from build123d import *

# Parameters (mm, degrees)
SKETCH1_R           = 1.75
BOSS_EXTRUDE1_DEPTH = 8
SKETCH2_R           = 3
CUT_EXTRUDE1_DEPTH  = 1.4
CUT_EXTRUDE2_DEPTH  = 59.268773799
FILLET1_R           = 2
CHAMFER1_SIZE       = 1
SKETCH4_R           = 4.541609358
CUT_EXTRUDE3_DEPTH  = 59.268773799
CHAMFER2_SIZE       = 2


with BuildPart() as part:
    # Sketch1 → Boss-Extrude1 (new body)
    with BuildSketch(Plane(origin=(0, 0, 0), x_dir=(1, 0, 0), z_dir=(0, 1, 0))):
        with BuildLine():
            Line((4.375, 16.94430214), (51.25, 4.841229183))
            ThreePointArc((51.25, 4.841229183), (55, 0), (51.25, -4.841229183))
            Line((51.25, -4.841229183), (4.375, -16.94430214))
            ThreePointArc((4.375, -16.94430214), (-17.5, 0), (4.375, 16.94430214))
        make_face()
        with Locations(Location((6.75, 11.691342951, 0), (0, 0, 270))):
            Circle(SKETCH1_R, mode=Mode.SUBTRACT)
        with Locations(Location((-13.5, 0, 0), (0, 0, 270))):
            Circle(SKETCH1_R, mode=Mode.SUBTRACT)
        with Locations(Location((6.75, -11.691342951, 0), (0, 0, 270))):
            Circle(SKETCH1_R, mode=Mode.SUBTRACT)
    extrude(amount=BOSS_EXTRUDE1_DEPTH)

    # Sketch2 → Cut-Extrude1 (cut)
    with BuildSketch(Plane(origin=(0, 8, 0), x_dir=(1, 0, 0), z_dir=(0, 1, 0))):
        with Locations(Location((6.75, -11.691342951, 0), (0, 0, 270))):
            Circle(SKETCH2_R)
        with Locations(Location((6.75, 11.691342951, 0), (0, 0, 270))):
            Circle(SKETCH2_R)
        with Locations(Location((-13.5, 0, 0), (0, 0, 270))):
            Circle(SKETCH2_R)
    extrude(amount=-CUT_EXTRUDE1_DEPTH, mode=Mode.SUBTRACT)

    # Sketch3 → Cut-Extrude2 (cut, through all)
    with BuildSketch(Plane(origin=(0, 8, 0), x_dir=(1, 0, 0), z_dir=(0, 1, 0))):
        with BuildLine():
            Line((21.175820833, -6.4095755), (46, 0))
            Line((46, 0), (21.175820833, 6.4095755))
            ThreePointArc((21.175820833, 6.4095755), (22.124602732, 0), (21.175820833, -6.4095755))
        make_face()
    extrude(amount=-CUT_EXTRUDE2_DEPTH, mode=Mode.SUBTRACT)

    # Fillet1
    fillet1_edges = [part.edges().sort_by_distance(p)[0] for p in [
        (21.175820833, 4, 6.4095755),
        (21.175820833, 4, -6.4095755),
        (46, 4, 0),
    ]]
    fillet(fillet1_edges, radius=FILLET1_R)

    # Chamfer1
    chamfer1_edges = [part.edges().sort_by_distance(p)[0] for p in [
        (6.75, 6.6, 8.691342951),
        (6.75, 6.6, -14.691342951),
        (-13.5, 6.6, -3),
    ]]
    chamfer(chamfer1_edges, length=CHAMFER1_SIZE)

    # Sketch4 → Cut-Extrude3 (cut, through all)
    with BuildSketch(Plane(origin=(0, 8, 0), x_dir=(1, 0, 0), z_dir=(0, 1, 0))):
        with Locations(Location((0, 0, 0), (0, 0, 270))):
            Circle(SKETCH4_R)
    extrude(amount=-CUT_EXTRUDE3_DEPTH, mode=Mode.SUBTRACT)

    # Chamfer2
    # the kernel refuses this chamfer: 2 mm, written as the material it takes off along each edge
    with BuildSketch(Plane(origin=(38, 0, 0), x_dir=(0.25, 0, 0.9682458365518543), z_dir=(-0.9682458365518543, 0, 0.25))) as chamfer2_piece_1:
        Polygon((2 + CHAMFER2_SIZE, 0), (2, CHAMFER2_SIZE), (2, 0), align=None)
    revolve(axis=Axis((38, 0, 0), (0, 1, 0)), revolution_arc=151.044975628, mode=Mode.SUBTRACT)
    with BuildSketch(Plane(origin=(24.346197065, 0, -5.590987877), x_dir=(0.24990547922782413, -0.027495876610586372, -0.9678797591753465), z_dir=(0.9682458365518543, 0, 0.24999999999999997)), Plane(origin=(38.5, 0, 1.936491673), x_dir=(0.2499054792278243, -0.027495876610585942, 0.9678797591753466), z_dir=(-0.9682458365518543, 0, 0.2500000000000001)), Plane(origin=(38.5, 8, -1.936491673), x_dir=(0.24990547922782413, 0.027495876610586497, -0.9678797591753466), z_dir=(-0.9682458365518543, 0, -0.24999999999999997)), Plane(origin=(24.346197065, 8, 5.590987877), x_dir=(0.2499054792278243, 0.02749587661058648, 0.9678797591753466), z_dir=(0.9682458365518543, 0, -0.2500000000000001))) as chamfer2_piece_2:
        Polygon((CHAMFER2_SIZE * 0.999621916911, CHAMFER2_SIZE * 0.0274958766106), (-CHAMFER2_SIZE * 0.0274958766106, CHAMFER2_SIZE * 0.999621916911), (0, 0), align=None)
    extrude(amount=14.617984814, mode=Mode.SUBTRACT)
    with BuildSketch(Plane(origin=(23.846197065, 0, -3.654496203), x_dir=(-0.9884596787014585, 0, 0.15148420241533292), z_dir=(0.15148420241533292, 0, 0.9884596787014585))) as chamfer2_piece_3:
        Polygon((2 + CHAMFER2_SIZE, 0), (2, -CHAMFER2_SIZE), (2, 0), align=None)
    revolve(axis=Axis((23.846197065, 0, -3.654496203), (0, -1, 0)), revolution_arc=113.190460245, mode=Mode.SUBTRACT)
    with BuildSketch(Plane(origin=(23.846197065, 0, 3.654496203), x_dir=(0.25000000000000006, 0, 0.9682458365518543), z_dir=(0.9682458365518543, 0, -0.25000000000000006))) as chamfer2_piece_4:
        Polygon((2 + CHAMFER2_SIZE, 0), (2, -CHAMFER2_SIZE), (2, 0), align=None)
    revolve(axis=Axis((23.846197065, 0, 3.654496203), (0, -1, 0)), revolution_arc=113.190460245, mode=Mode.SUBTRACT)
    with BuildSketch(Plane(origin=(0, 0, 0), x_dir=(0.988459678701458, 0, 0.151484202415335), z_dir=(-0.151484202415335, 0, 0.988459678701458))) as chamfer2_piece_5:
        Polygon((22.124602732 - CHAMFER2_SIZE, 0), (22.124602732, CHAMFER2_SIZE), (22.124602732, 0), align=None)
    revolve(axis=Axis((0, 0, 0), (0, 1, 0)), revolution_arc=17.425896117, mode=Mode.SUBTRACT)
    with BuildSketch(Plane(origin=(23.846197065, 8, -3.654496203), x_dir=(-0.9884596787014583, 0, 0.15148420241533467), z_dir=(0.15148420241533467, 0, 0.9884596787014583))) as chamfer2_piece_6:
        Polygon((2 + CHAMFER2_SIZE, 0), (2, CHAMFER2_SIZE), (2, 0), align=None)
    revolve(axis=Axis((23.846197065, 8, -3.654496203), (0, -1, 0)), revolution_arc=113.190460245, mode=Mode.SUBTRACT)
    with BuildSketch(Plane(origin=(0, 8, 0), x_dir=(0.9884596787014582, 0, -0.1514842024153346), z_dir=(-0.1514842024153346, 0, -0.9884596787014582))) as chamfer2_piece_7:
        Polygon((22.124602732 - CHAMFER2_SIZE, 0), (22.124602732, CHAMFER2_SIZE), (22.124602732, 0), align=None)
    revolve(axis=Axis((0, 8, 0), (0, -1, 0)), revolution_arc=17.425896117, mode=Mode.SUBTRACT)
    with BuildSketch(Plane(origin=(23.846197065, 8, 3.654496203), x_dir=(0.25000000000000006, 0, 0.9682458365518543), z_dir=(0.9682458365518543, 0, -0.25000000000000006))) as chamfer2_piece_8:
        Polygon((2 + CHAMFER2_SIZE, 0), (2, CHAMFER2_SIZE), (2, 0), align=None)
    revolve(axis=Axis((23.846197065, 8, 3.654496203), (0, -1, 0)), revolution_arc=113.190460245, mode=Mode.SUBTRACT)
    with BuildSketch(Plane(origin=(38, 8, 0), x_dir=(0.25, 0, 0.9682458365518543), z_dir=(-0.9682458365518543, 0, 0.25))) as chamfer2_piece_9:
        Polygon((2 + CHAMFER2_SIZE, 0), (2, -CHAMFER2_SIZE), (2, 0), align=None)
    revolve(axis=Axis((38, 8, 0), (0, 1, 0)), revolution_arc=151.044975628, mode=Mode.SUBTRACT)
    with BuildSketch(Plane(origin=(4.375, 0, -16.94430214), x_dir=(-0.24990547922782413, -0.027495876610586365, 0.9678797591753465), z_dir=(0.9682458365518543, 0, 0.24999999999999997)), Plane(origin=(51.25, 0, 4.841229183), x_dir=(-0.2499054792278242, -0.027495876610586348, -0.9678797591753466), z_dir=(-0.9682458365518543, 0, 0.24999999999999997))) as chamfer2_piece_10:
        Polygon((CHAMFER2_SIZE * 0.999621916911, -CHAMFER2_SIZE * 0.0274958766106), (-CHAMFER2_SIZE * 0.0274958766106, -CHAMFER2_SIZE * 0.999621916911), (0, 0), align=None)
    extrude(amount=48.412291828, mode=Mode.SUBTRACT)
    with BuildSketch(Plane(origin=(0, 0, 0), x_dir=(0.24999999999999994, 0, 0.9682458365518543), z_dir=(0.9682458365518543, 0, -0.24999999999999994))) as chamfer2_piece_11:
        Polygon((17.5 - CHAMFER2_SIZE, 0), (17.5, -CHAMFER2_SIZE), (17.5, 0), align=None)
    revolve(axis=Axis((0, 0, 0), (0, -1, 0)), revolution_arc=208.955024372, mode=Mode.SUBTRACT)
    with BuildSketch(Plane(origin=(50, 0, 0), x_dir=(0.25000000000000105, 0, -0.9682458365518539), z_dir=(-0.9682458365518539, 0, -0.25000000000000105))) as chamfer2_piece_12:
        Polygon((5 - CHAMFER2_SIZE, 0), (5, -CHAMFER2_SIZE), (5, 0), align=None)
    revolve(axis=Axis((50, 0, 0), (0, -1, 0)), revolution_arc=151.044975628, mode=Mode.SUBTRACT)
    with BuildSketch(Plane(origin=(50, 8, 0), x_dir=(0.25000000000000105, 0, -0.9682458365518539), z_dir=(-0.9682458365518539, 0, -0.25000000000000105))) as chamfer2_piece_13:
        Polygon((5 - CHAMFER2_SIZE, 0), (5, CHAMFER2_SIZE), (5, 0), align=None)
    revolve(axis=Axis((50, 8, 0), (0, -1, 0)), revolution_arc=151.044975628, mode=Mode.SUBTRACT)
    with BuildSketch(Plane(origin=(0, 0, 0), x_dir=(0, 0, 1), z_dir=(-1, 0, 0))) as chamfer2_piece_14:
        Polygon((4.541609358 + CHAMFER2_SIZE, 0), (4.541609358, CHAMFER2_SIZE), (4.541609358, 0), align=None)
    revolve(axis=Axis((0, 0, 0), (0, 1, 0)), mode=Mode.SUBTRACT)
    with BuildSketch(Plane(origin=(0, 8, 0), x_dir=(0, 0, 1), z_dir=(-1, 0, 0))) as chamfer2_piece_15:
        Polygon((4.541609358 + CHAMFER2_SIZE, 0), (4.541609358, -CHAMFER2_SIZE), (4.541609358, 0), align=None)
    revolve(axis=Axis((0, 8, 0), (0, 1, 0)), mode=Mode.SUBTRACT)
    with BuildSketch(Plane(origin=(4.375, 8, -16.94430214), x_dir=(-0.24990547922782413, 0.02749587661058648, 0.9678797591753465), z_dir=(0.9682458365518543, 0, 0.24999999999999997)), Plane(origin=(51.25, 8, 4.841229183), x_dir=(-0.2499054792278242, 0.027495876610586473, -0.9678797591753466), z_dir=(-0.9682458365518543, 0, 0.24999999999999997))) as chamfer2_piece_16:
        Polygon((CHAMFER2_SIZE * 0.999621916911, CHAMFER2_SIZE * 0.0274958766106), (-CHAMFER2_SIZE * 0.0274958766106, CHAMFER2_SIZE * 0.999621916911), (0, 0), align=None)
    extrude(amount=48.412291828, mode=Mode.SUBTRACT)
    with BuildSketch(Plane(origin=(0, 8, 0), x_dir=(0.24999999999999994, 0, 0.9682458365518543), z_dir=(0.9682458365518543, 0, -0.24999999999999994))) as chamfer2_piece_17:
        Polygon((17.5 - CHAMFER2_SIZE, 0), (17.5, CHAMFER2_SIZE), (17.5, 0), align=None)
    revolve(axis=Axis((0, 8, 0), (0, -1, 0)), revolution_arc=208.955024372, mode=Mode.SUBTRACT)


solid = part.part
The model under review builds one solid part; all positions refer to its coordinate system, in mm. A direction names the side the tool comes from. Give positions to 0.01 mm unless a question says otherwise; leave off trailing zeros. Write each loop counter-clockwise with the first axis right and the second up, starting at its lowest first coordinate (ties: lowest second). Pieces come first, ordered by that corner, then holes.
1. For P1, Ø3, axis at x = 36.5, y = 5, coming from the +Z side; P2, Ø10.5, axis at x = 0, z = 0, coming from the +Y side; P3, Ø1.5, axis at y = 6.5, z = 13.5, coming from the -X side, all flat-tipped, find the tip position at first contact; note any pin that passes through.
2. Add section C-C, the plane x = 45.5. Write out the cut boundary in (y, z).
3. Add section A-A, the plane z = 0. Count the separate pieces of the cut face and the enclosed holes in it, plus the area to 3 significant figures.
4. Tool access review of faces 1 (the flat face through (31.52, 4.03, -3.74)), 2 (the flat face through (12, 8, 0)), 3 (the cylindrical face through (-10.5, 7.8, 0.1)): name each direction out of +Z, -Z, +X, -X, +Y, -Y from which nothing blocks a thin tool from reaching the whole face with its end or side.
5. Draft analysis for pull direction X (two halves, no side actions). For faces 4 (the cylindrical face through (55, 4, 0)), 5 (the flat face through (12, 0, 0)), 6 (the conical face through (41, 1, 0)), state which applies: +X half, -X half, draft (parallel to the pull), parting line (faces both ways), or undercut.
6. Add section D-D, the plane x = 16. Write out the cut boundary in (y, z), plus the area to 3 significant figures.
7. Add section B-B, the plane x = 0. Write out the cut boundary in (y, z), plus the area to 3 significant figures.
8. Wall thickness on L1, parallel to Z at x = 6.75, y = 4.5; L2, parallel to Z at x = 32, y = 7; L3, parallel to Z at x = 28, y = 5.25: over which ranges is each line inside the solid? List them lowest first.
Worked answers:
1. P1: stops at z = 9.04
1. P2: stops at y = 6.71
1. P3: stops at x = -11.78
2. outline: (0, -4.26) - (2, -6.33) - (6, -6.33) - (8, -4.26) - (8, 4.26) - (6, 6.33) - (2, 6.33) - (0, 4.26) - close
3. separate pieces: 4
3. enclosed holes: 0
3. area: 310 mm2
4. face 1: +Y, -Y
4. face 2: +Z, -Z, +X, -X, +Y
4. face 3: +Y
5. face 4: +X half
5. face 5: draft
5. face 6: undercut
6. outline: (0, -11.88) - (2, -13.94) - (6, -13.94) - (8, -11.88) - (8, 11.88) - (6, 13.94) - (2, 13.94) - (0, 11.88) - close
6. area: 215 mm2
7. outline: (0, -15.5) - (2, -17.5) - (6, -17.5) - (8, -15.5) - (8, -6.54) - (6, -4.54) - (2, -4.54) - (0, -6.54) - close; (0, 6.54) - (2, 4.54) - (6, 4.54) - (8, 6.54) - (8, 15.5) - (6, 17.5) - (2, 17.5) - (0, 15.5) - close
7. area: 191 mm2
8. L1: z = -16.33 to -13.44, -9.94 to 9.94, 13.44 to 16.33
8. L2: z = -8.78 to -4.65, 4.65 to 8.78
8. L3: z = -10.84 to -4.65, 4.65 to 10.84
